from build123d import *

# Parameters (mm, degrees)
SKETCH1_W                                       = 12
SKETCH1_H                                       = 8
BOSS_EXTRUDE1_DEPTH                             = 500
CSK_FOR_M3_FLAT_HEAD_MACHINE_SCREW1_D           = 3.4
CSK_FOR_M3_FLAT_HEAD_MACHINE_SCREW1_CSINK_D     = 6.3
CSK_FOR_M3_FLAT_HEAD_MACHINE_SCREW1_CSINK_ANGLE = 90
LPATTERN1_COUNT                                 = 20
LPATTERN1_PITCH                                 = 25


with BuildPart() as part:
    # Sketch1 → Boss-Extrude1 (new body)
    with BuildSketch(Plane(origin=(0, 0, 0), x_dir=(0, 0, -1), z_dir=(1, 0, 0))):
        Rectangle(SKETCH1_W, SKETCH1_H)
    extrude(amount=BOSS_EXTRUDE1_DEPTH)

    # CSK for M3 Flat Head Machine Screw1 (through all)
    with Locations(Plane(origin=(0, 4, 0), x_dir=(1, 0, 0), z_dir=(0, 1, 0))):
        with Locations((10, 0)):
            csk_for_m3_flat_head_machine_screw1 = CounterSinkHole(CSK_FOR_M3_FLAT_HEAD_MACHINE_SCREW1_D / 2, CSK_FOR_M3_FLAT_HEAD_MACHINE_SCREW1_CSINK_D / 2, counter_sink_angle=CSK_FOR_M3_FLAT_HEAD_MACHINE_SCREW1_CSINK_ANGLE)

    # LPattern1: CSK for M3 Flat Head Machine Screw1 ×20
    with Locations(*[(i * LPATTERN1_PITCH, 0, 0) for i in range(1, LPATTERN1_COUNT)]):
        add(csk_for_m3_flat_head_machine_screw1, mode=Mode.SUBTRACT)


solid = part.part
CAD build for the part. Positions are in the model's coordinates, mm. Give positions to 0.01 mm unless a question says otherwise; leave off trailing zeros. Put each result on its own line as item: value. Start each with the question number.
(1) Band-saw the part on A-A, the plane y = -1.75. Give the number of separate pieces and of enclosed holes in the cut face, and give its area (3 significant figures).
(2) Probe L1, parallel to Z at x = 410, y = 0.75; L2, parallel to Z at x = 209.5, y = 1.5; L3, parallel to Y at x = 461.5, z = -1.5. List the from-to ranges inside material, lowest first.
(3) Flat gauge pins, fed straight in: pin 1 Ø3 at (x, z) = (410, 0) entering from -Y; pin 2 Ø4.5 at (x, z) = (310, 0) entering from +Y; pin 3 Ø4 at (x, z) = (185, 0) entering from +Y; pin 4 Ø5.5 at (x, z) = (110, 0) entering from +Y. Where does each tip first touch, or does it go through?
Response values:
1. separate pieces: 1
1. enclosed holes: 20
1. area: 5,820 mm2
2. L1: z = -6 to -1.7, 1.7 to 6
2. L2: z = -6 to -1.62, 1.62 to 6
2. L3: y = -4 to 2.97
3. pin 1: passes through
3. pin 2: stops at y = 3.1
3. pin 3: stops at y = 2.85
3. pin 4: stops at y = 3.6
